Design review of the part built by this model. Coordinates are the model's own, in mm. A direction names the side the tool comes from. Give positions to 0.01 mm unless a question says otherwise; leave off trailing zeros. Loops run counter-clockwise (first coordinate to the right, second up) from the corner with the lowest first, then second, coordinate; pieces in that order, holes last. Notation, with made-up numbers: (20, -23) - (31, -23) arc R6 cw to (31, -13) - close; hole circle Ø3 at (-2.75, -8.75). An arc over 180 degrees is marked (long way). Write each question's results on one line, items separated by ' | '.
```python
from build123d import *

# Parameters (mm, degrees)
SKETCH1_R                    = 11
BOSS_EXTRUDE1_DEPTH          = 100
FILLET1_R                    = 8
SKETCH2_R                    = 4.1
SKETCH2_R_2                  = 6
CUT_EXTRUDE1_DEPTH           = 10
BOSS_EXTRUDE2_START          = 20
SKETCH3_R                    = 4.1
SKETCH3_R_2                  = 6
BOSS_EXTRUDE2_DEPTH          = 20
FILLET2_R                    = 3
CUT_EXTRUDE_THIN1_DEPTH      = 183.94618817
CUT_EXTRUDE_THIN1_DEPTH_BACK = 20
CUT_EXTRUDE_THIN2_DEPTH      = 163.832913644
CUT_EXTRUDE_THIN2_DEPTH_BACK = 20
FILLET3_R                    = 3
CUT_EXTRUDE2_DEPTH           = 161.472919104
CUT_EXTRUDE2_DEPTH_BACK      = 161.472919104
SKETCH6_R                    = 2.25
CUT_EXTRUDE3_DEPTH           = 3
CUT_EXTRUDE4_DEPTH           = 25
CUT_EXTRUDE5_START           = 25
CUT_EXTRUDE5_DEPTH           = 25


with BuildPart() as part:
    # Sketch1 → Boss-Extrude1 (new body)
    with BuildSketch(Plane(origin=(0, 0, 0), x_dir=(1, 0, 0), z_dir=(0, 1, 0))):
        with BuildLine():
            Line((137.460581558, -14.5), (119.460581558, -14.5))
            Line((119.460581558, -14.5), (119.460581558, 10.5))
            Line((119.460581558, 10.5), (-24.539418442, 10.5))
            Line((-24.539418442, 10.5), (-24.539418442, -14.5))
            Line((-24.539418442, -14.5), (-42.539418442, -14.5))
            ThreePointArc((-42.539418442, -14.5), (-56.539418442, -0.5), (-42.539418442, 13.5))
            Line((-42.539418442, 13.5), (137.460581558, 13.5))
            ThreePointArc((137.460581558, 13.5), (151.460581558, -0.5), (137.460581558, -14.5))
        make_face()
        with Locations(Location((-42.539418442, -0.5, 0), (0, 0, 270))):
            Circle(SKETCH1_R, mode=Mode.SUBTRACT)
        with Locations(Location((137.460581558, -0.5, 0), (0, 0, 270))):
            Circle(SKETCH1_R, mode=Mode.SUBTRACT)
    extrude(amount=BOSS_EXTRUDE1_DEPTH)

    # Fillet1
    fillet1_edges = [part.edges().sort_by_distance(p)[0] for p in [
        (119.460581558, 50, 14.5),
        (119.460581558, 50, -10.5),
        (-24.539418442, 50, -10.5),
        (-24.539418442, 50, 14.5),
    ]]
    fillet(fillet1_edges, radius=FILLET1_R)

    # Sketch2 → Cut-Extrude1 (cut)
    with BuildSketch(Plane.XY.offset(-10.5)):
        with Locations((12.460581558, 50)):
            Circle(SKETCH2_R)
        with Locations((82.460581558, 50)):
            Circle(SKETCH2_R)
        with Locations((47.460581558, 50)):
            Circle(SKETCH2_R_2)
    extrude(amount=-CUT_EXTRUDE1_DEPTH, mode=Mode.SUBTRACT)

    # Sketch3 → Boss-Extrude2 (add)
    with BuildSketch(Plane.XY.offset(-10.5).offset(BOSS_EXTRUDE2_START)):
        Polygon((12.460581558, 58), (82.460581558, 58), (124.149440998, 58), (124.149440998, 42), (82.460581558, 42), (12.460581558, 42), (-28.8662965, 42), (-28.8662965, 58), (-16.539418442, 58), align=None)
        with Locations((12.460581558, 50)):
            Circle(SKETCH3_R, mode=Mode.SUBTRACT)
        with Locations((82.460581558, 50)):
            Circle(SKETCH3_R, mode=Mode.SUBTRACT)
        with Locations((47.460581558, 50)):
            Circle(SKETCH3_R_2, mode=Mode.SUBTRACT)
    extrude(amount=-BOSS_EXTRUDE2_DEPTH)

    # Fillet2
    fillet2_edges = [part.edges().sort_by_distance(p)[0] for p in [
        (-24.686725022, 58, 8.0281381),
        (-24.686725022, 42, 8.0281381),
        (47.460581558, 42, -10.5),
        (117.117435807, 42, -8.156854249),
        (119.460581558, 42, 2),
        (-24.539418442, 42, 2),
        (-22.196272692, 42, -8.156854249),
        (119.607888138, 42, 8.0281381),
        (119.460581558, 58, 2),
        (117.117435807, 58, -8.156854249),
        (47.460581558, 58, -10.5),
        (-22.196272692, 58, -8.156854249),
        (-24.539418442, 58, 2),
        (119.607888138, 58, 8.0281381),
    ]]
    fillet(fillet2_edges, radius=FILLET2_R)

    # Sketch4 → Cut-Extrude-Thin1 (cut, two sides: drawn at the far end of the back side and taken through both)
    with BuildSketch(Plane.XY.offset(9.5).offset(-CUT_EXTRUDE_THIN1_DEPTH_BACK)):
        Polygon((92.460581558, 51), (47.460581558, 51), (2.460581558, 51), (2.460581558, 49), (47.460581558, 49), (92.460581558, 49), align=None)
    extrude(amount=CUT_EXTRUDE_THIN1_DEPTH + CUT_EXTRUDE_THIN1_DEPTH_BACK, mode=Mode.SUBTRACT)

    # Sketch5 → Cut-Extrude-Thin2 (cut, two sides: drawn at the far end of the back side and taken through both)
    with BuildSketch(Plane(origin=(0, 42, 0), x_dir=(-1, 0, 0), z_dir=(0, -1, 0)).offset(-CUT_EXTRUDE_THIN2_DEPTH_BACK)):
        Polygon((-2.460581558, 7.5), (-47.460581558, 7.5), (-92.460581558, 7.5), (-92.460581558, 10.5), (-47.460581558, 10.5), (-2.460581558, 10.5), align=None)
    extrude(amount=CUT_EXTRUDE_THIN2_DEPTH + CUT_EXTRUDE_THIN2_DEPTH_BACK, mode=Mode.SUBTRACT)

    # Fillet3
    fillet3_edges = [part.edges().sort_by_distance(p)[0] for p in [
        (92.460581558, 50, -10.5),
        (2.460581558, 50, -10.5),
    ]]
    fillet(fillet3_edges, radius=FILLET3_R - 0.0001)  # a hair under: the kernel refuses the full size

    # Sketch6 → Cut-Extrude2 (cut, two sides: drawn at the far end of the back side and taken through both)
    with BuildSketch(Plane(origin=(0, 49, 0), x_dir=(1, 0, 0), z_dir=(0, 1, 0)).offset(-CUT_EXTRUDE2_DEPTH_BACK)):
        with Locations(Location((28.990631201, -1, 0), (0, 0, 270))):
            Circle(SKETCH6_R)
        with Locations(Location((65.930531914, -1, 0), (0, 0, 270))):
            Circle(SKETCH6_R)
    extrude(amount=CUT_EXTRUDE2_DEPTH + CUT_EXTRUDE2_DEPTH_BACK, mode=Mode.SUBTRACT)

    # Sketch7 → Cut-Extrude3 (cut)
    with BuildSketch(Plane(origin=(0, 58, 0), x_dir=(1, 0, 0), z_dir=(0, 1, 0))):
        Polygon((33.150591825, -0.026315789), (30.227376252, 3.089473684), (26.067415628, 2.115789474), (24.830670578, -1.973684211), (27.753886151, -5.089473684), (31.913846775, -4.115789474), align=None)
        Polygon((70.090492538, -0.026315789), (67.167276964, 3.089473684), (63.007316341, 2.115789474), (61.77057129, -1.973684211), (64.693786864, -5.089473684), (68.853747488, -4.115789474), align=None)
    extrude(amount=-CUT_EXTRUDE3_DEPTH, mode=Mode.SUBTRACT)

    # Sketch8 → Cut-Extrude4 (cut)
    with BuildSketch(Plane(origin=(0, 100, 0), x_dir=(1, 0, 0), z_dir=(0, 1, 0))):
        with BuildLine():
            Line((119.460581558, 2.5), (119.460581558, -6.5))
            ThreePointArc((119.460581558, -6.5), (121.803727308, -12.156854249), (127.460581558, -14.5))
            Line((127.460581558, -14.5), (137.460581558, -14.5))
            ThreePointArc((137.460581558, -14.5), (151.460581558, -0.5), (137.460581558, 13.5))
            Line((137.460581558, 13.5), (-42.539418442, 13.5))
            ThreePointArc((-42.539418442, 13.5), (-56.539418442, -0.5), (-42.539418442, -14.5))
            Line((-42.539418442, -14.5), (-32.539418442, -14.5))
            ThreePointArc((-32.539418442, -14.5), (-26.882564193, -12.156854249), (-24.539418442, -6.5))
            Line((-24.539418442, -6.5), (-24.539418442, 2.5))
            ThreePointArc((-24.539418442, 2.5), (-22.196272692, 8.156854249), (-16.539418442, 10.5))
            Line((-16.539418442, 10.5), (111.460581558, 10.5))
            ThreePointArc((111.460581558, 10.5), (117.117435807, 8.156854249), (119.460581558, 2.5))
        make_face()
    extrude(amount=-CUT_EXTRUDE4_DEPTH, mode=Mode.SUBTRACT)

    # Sketch9 → Cut-Extrude5 (cut)
    with BuildSketch(Plane(origin=(0, 0, 0), x_dir=(1, 0, 0), z_dir=(0, 1, 0)).offset(CUT_EXTRUDE5_START)):
        with BuildLine():
            Line((127.460581558, -14.5), (137.460581558, -14.5))
            ThreePointArc((137.460581558, -14.5), (151.460581558, -0.5), (137.460581558, 13.5))
            Line((137.460581558, 13.5), (-42.539418442, 13.5))
            ThreePointArc((-42.539418442, 13.5), (-56.539418442, -0.5), (-42.539418442, -14.5))
            Line((-42.539418442, -14.5), (-32.539418442, -14.5))
            ThreePointArc((-32.539418442, -14.5), (-26.882564193, -12.156854249), (-24.539418442, -6.5))
            Line((-24.539418442, -6.5), (-24.539418442, 2.5))
            ThreePointArc((-24.539418442, 2.5), (-22.196272692, 8.156854249), (-16.539418442, 10.5))
            Line((-16.539418442, 10.5), (111.460581558, 10.5))
            ThreePointArc((111.460581558, 10.5), (117.117435807, 8.156854249), (119.460581558, 2.5))
            Line((119.460581558, 2.5), (119.460581558, -6.5))
            ThreePointArc((119.460581558, -6.5), (121.803727308, -12.156854249), (127.460581558, -14.5))
        make_face()
    extrude(amount=-CUT_EXTRUDE5_DEPTH, mode=Mode.SUBTRACT)


solid = part.part
```
Item 1: Wall thickness on probe 1 along X at (y, z) = (60.5, 0.5); probe 2 along X at (y, z) = (61, 1); probe 3 along Y at (x, z) = (8, 6.25): over which ranges is each line inside the solid? List them lowest first.
Output values:
probe 1: x = -56.54 to -53.54, -31.54 to -24.5, 119.42 to 126.46, 148.46 to 151.46 | probe 2: x = -56.53 to -53.53, -31.55 to -24.54, 119.46 to 126.47, 148.45 to 151.45 | probe 3: y = 42 to 49, 51 to 58
Item 2: We need section C-C on z = -5.5. Give the number of separate pieces and of enclosed holes in the cut face, then the cut area to 3 significant figures.
Output values:
separate pieces: 3 | enclosed holes: 1 | area: 3,230 mm²
Item 3: Clearance check with flat-ended pins moving along their axes: P1, Ø5, axis at x = 92.5, y = 37, coming from the +Z side; P2, Ø24, axis at x = 56, y = 44.5, coming from the +Z side; P3, Ø5, axis at x = 77.5, z = 2.5, coming from the -Y side. State where each tip first meets the part, or that it passes through.
Output values:
P1: stops at z = -10.46 | P2: stops at z = 9.5 | P3: stops at y = 42
Item 4: Tool access review of faces 4 (the face through (119.461, 68, 2)), 5 (the face through (12.5, 54.1, 1.1)), 6 (the face through (63, 49, 1)): name each direction out of +Z, -Z, +X, -X, +Y, -Y from which nothing blocks a thin tool from reaching the whole face with its end or side.
Output values:
face 4: +Z, +Y | face 5: +Z, -Z | face 6: +Z
Item 5: We need section B-B on x = 37. Give the boundary of the cut face in (y, z).
Output values:
outline: (25, -13.5) - (75, -13.5) - (75, -10.5) - (25, -10.5) - close; (42, -7.5) - (49, -7.5) - (49, 9.5) - (42, 9.5) - close; (51, -7.5) - (58, -7.5) - (58, 9.5) - (51, 9.5) - close
Item 6: We need section A-A on y = 67. Give the boundary of the cut face in (x, z).
Output values:
outline: (-42.54, -13.5) - (137.46, -13.5) arc R14 ccw to (137.46, 14.5) - (127.46, 14.5) arc R8 ccw to (119.46, 6.5) - (119.46, -2.5) arc R8 cw to (111.46, -10.5) - (-16.54, -10.5) arc R8 cw to (-24.54, -2.5) - (-24.54, 6.5) arc R8 ccw to (-32.54, 14.5) - (-42.54, 14.5) arc R14 ccw to start; hole circle Ø22 at (-42.54, 0.5); hole circle Ø22 at (137.46, 0.5)
Item 7: Draft analysis for pull direction X (two halves, no side actions). For faces 1 (the face through (-24.539, 32, 2)), 2 (the face through (-37, 50, 14.5)), 3 (the face through (63.934, 52.972, 2.038)), state which applies: +X half, -X half, draft (parallel to the pull), parting line (faces both ways), or undercut.
Output values:
face 1: undercut | face 2: draft | face 3: undercut
